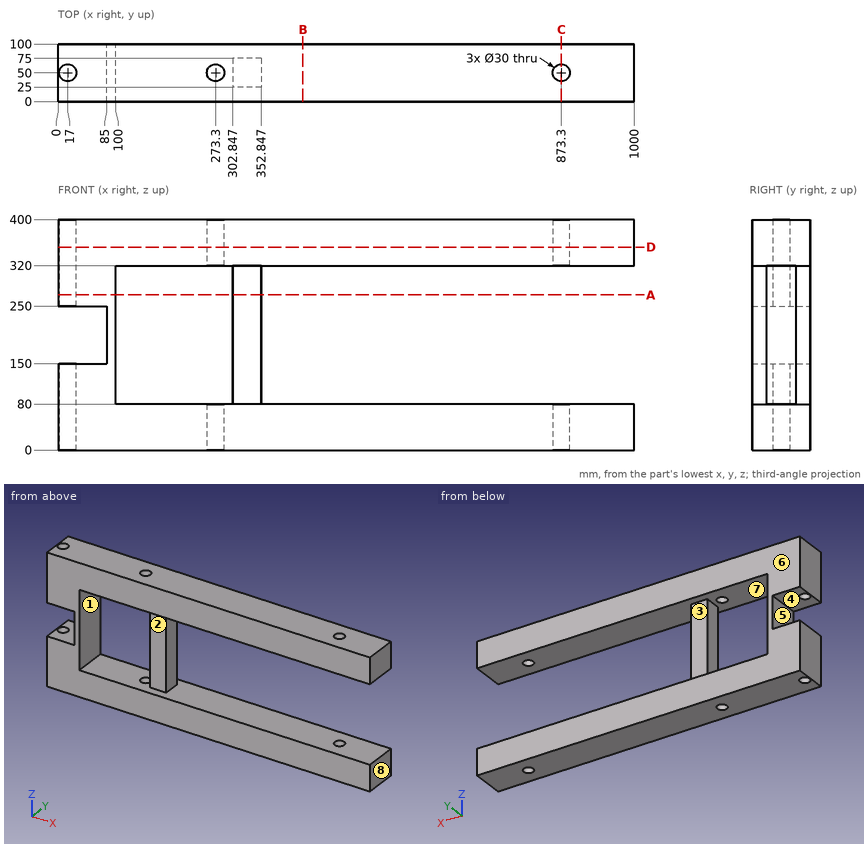
Could you check a few things on this drawing? It's one solid part, dimensions in mm from its lowest x, y, z. A direction names the side the tool comes from. Round coordinates to 2 decimals unless told otherwise and drop trailing zeros. Loops run counter-clockwise (first coordinate to the right, second up) from the corner with the lowest first, then second, coordinate; pieces in that order, holes last.
Q1. For P1, Ø15, axis at x = 324.5, z = 152, coming from the -Y side; P2, Ø3, axis at y = 20, z = 261.5, coming from the +X side, each with a flat end and sliding along its axis, tell me the tip position at first contact or that it passes through.
Q2. I want a section at A-A (z = 269.5). Write out the boundary of the cut face in (x, y), and give its area (3 significant figures).
Q3. I want a section at B-B (x = 425). Write out the boundary of the cut face in (y, z).
Q4. I want a section at D-D (z = 352.5). Write out the boundary of the cut face in (x, y), and give its area (3 significant figures).
Q5. Please list where these lines run through material, in increasing order: L1, parallel to X at y = 50, z = 358.5; L2, parallel to Z at x = 185.5, y = 30; L3, parallel to Y at x = 873, z = 359.
Q6. I want a section at C-C (x = 873.3). Write out the boundary of the cut face in (y, z).
Q7. Thinking about a two-plate mould opening in X: for the marked faces 5, 6, 7 and 8, which applies, pulls with the +X half, pulls with the -X half, needs draft (parallel to the pull), parting line crosses it, or undercut?
Q8. On a 3-axis mill with a long thin cutter (end or side, diameter ignored), from which of +Z, -Z, +X, -X, +Y, -Y can I reach the whole of each face in a straight line? I mean the marked faces 1, 2, 3 and 4. Say none if no direction works.
Answer below:
1. P1: stops at y = 25
1. P2: stops at x = 100
2. outline: (0, 0) - (100, 0) - (100, 100) - (0, 100) - close; (302.85, 25) - (352.85, 25) - (352.85, 75) - (302.85, 75) - close; hole circle Ø30 at (17, 50)
2. area: 11,800 mm2
3. outline: (0, 0) - (100, 0) - (100, 80) - (0, 80) - close; (0, 320) - (100, 320) - (100, 400) - (0, 400) - close
4. outline: (0, 0) - (1000, 0) - (1000, 100) - (0, 100) - close; hole circle Ø30 at (17, 50); hole circle Ø30 at (273.3, 50); hole circle Ø30 at (873.3, 50)
4. area: 97,900 mm2
5. L1: x = 0 to 2, 32 to 258.3, 288.3 to 858.3, 888.3 to 1000
5. L2: z = 0 to 80, 320 to 400
5. L3: y = 0 to 35, 65 to 100
6. outline: (0, 0) - (35, 0) - (35, 80) - (0, 80) - close; (0, 320) - (35, 320) - (35, 400) - (0, 400) - close; (65, 0) - (100, 0) - (100, 80) - (65, 80) - close; (65, 320) - (100, 320) - (100, 400) - (65, 400) - close
7. face 5: pulls with the -X half
7. face 6: needs draft
7. face 7: undercut
7. face 8: pulls with the +X half
8. face 1: +Y, -Y
8. face 2: +X, -Y
8. face 3: +X, +Y
8. face 4: -X, +Y, -Y
